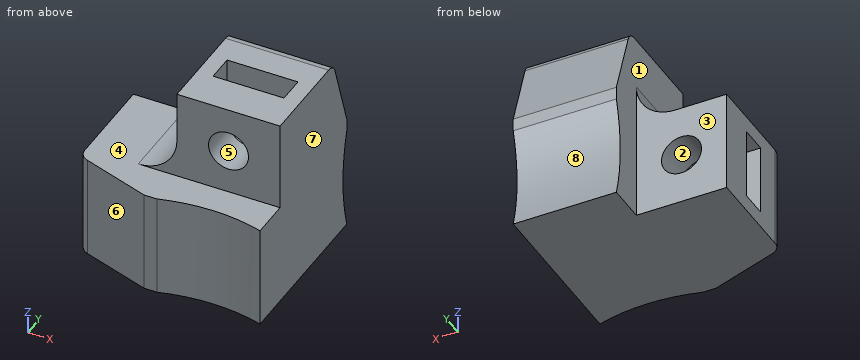
```python
from build123d import *

# Parameters (mm, degrees)
EXTRUDE002_DEPTH                          = 2.1
EXTRUDE002_ONTO_SKETCH006_ROLL_ANGLE      = 90
EXTRUDE001_DEPTH                          = 2.1
EXTRUDE001_ONTO_SKETCH005_ROLL_ANGLE      = 90
EXTRUDE001_ONTO_SKETCH005_PLACEMENT_ANGLE = 180
EXTRUDE_DEPTH                             = 8
SKETCH001_W                               = 8
SKETCH001_H                               = 10
PAD_DEPTH                                 = 7
POCKET_DEPTH                              = 8.001
SKETCH003_R                               = 1.55
POCKET001_DEPTH                           = 7
SKETCH004_R                               = 1.55
POCKET002_DEPTH                           = 7
CHAMFER_SIZE2                             = 2
CHAMFER_SIZE                              = 6
CHAMFER001_SIZE2                          = 6
CHAMFER001_SIZE                           = 2
FILLET_1_R                                = 3
FILLET_2_R                                = 1


with BuildPart() as extrude002:
    # Sketch006 as drawn → Extrude002 (new)
    with BuildSketch(Plane.XY):
        Polygon((4, 8.324574), (1.25, 9.912287), (1.25, 15), (6.75, 15), (6.75, 9.912287), align=None)
    extrude(amount=-EXTRUDE002_DEPTH)


with BuildPart() as extrude002_1:
    # Extrude002 onto Sketch006 roll: moved
    add(extrude002.part.rotate(Axis((0, 0, 0), (1, 0, 0)), EXTRUDE002_ONTO_SKETCH006_ROLL_ANGLE))


with BuildPart() as extrude002_2:
    # Extrude002 onto Sketch006 placement: moved
    add(extrude002_1.part.moved(Location((0, -7, 0))))


with BuildPart() as extrude002_3:
    # Extrude002 placement: moved
    add(extrude002_2.part.moved(Location((0, 3, 0))))


with BuildPart() as extrude001:
    # Sketch005 as drawn → Extrude001 (new)
    with BuildSketch(Plane.XY):
        Polygon((0.324574, 4), (1.912287, 6.75), (7, 6.75), (7, 1.25), (1.912287, 1.25), align=None)
    extrude(amount=-EXTRUDE001_DEPTH)


with BuildPart() as extrude001_1:
    # Extrude001 onto Sketch005 roll: moved
    add(extrude001.part.rotate(Axis((0, 0, 0), (1, 0, 0)), EXTRUDE001_ONTO_SKETCH005_ROLL_ANGLE))


with BuildPart() as extrude001_2:
    # Extrude001 onto Sketch005 placement: moved
    add(extrude001_1.part.rotate(Axis((0, 0, 0), (0, 0, 1)), EXTRUDE001_ONTO_SKETCH005_PLACEMENT_ANGLE))


with BuildPart() as extrude001_3:
    # Extrude001 placement: moved
    add(extrude001_2.part.moved(Location((0, -3, 0))))


with BuildPart() as fillet_body:
    # Sketch → Extrude (new body)
    with BuildSketch(Plane.XY):
        with BuildLine():
            Line((0, 0), (0, 3))
            Line((0, 3), (8, 3))
            Line((8, 3), (8, -10))
            ThreePointArc((8, -10), (4, -9.422859), (0, -10))
            Line((0, -10), (-7, -10))
            Line((-7, -10), (-7, 0))
            Line((-7, 0), (0, 0))
        make_face()
    extrude(amount=EXTRUDE_DEPTH)

    # Sketch001 → Pad (new body)
    with BuildSketch(Plane.XY.offset(8)):
        with Locations((4, -2)):
            Rectangle(SKETCH001_W, SKETCH001_H)
    extrude(amount=PAD_DEPTH)

    # Sketch002 → Pocket (cut, through all)
    with BuildSketch(Plane(origin=(0, 0, 0), x_dir=(0, -1, 0), z_dir=(-1, 0, 0))):
        with BuildLine():
            Line((-3, 0), (-3, 8))
            ThreePointArc((-3, 0), (-2.422859, 4), (-3, 8))
        make_face()
    extrude(amount=-POCKET_DEPTH, mode=Mode.SUBTRACT)

    # Sketch003 → Pocket001 (cut)
    with BuildSketch(Plane(origin=(0, 0, 0), x_dir=(-1, 0, 0), z_dir=(0, 1, 0))):
        with Locations((3.5, 4)):
            Circle(SKETCH003_R)
    extrude(amount=-POCKET001_DEPTH, mode=Mode.SUBTRACT)

    # Sketch004 → Pocket002 (cut)
    with BuildSketch(Plane.XZ.offset(7)):
        with Locations((4, 11.5)):
            Circle(SKETCH004_R)
    extrude(amount=-POCKET002_DEPTH, mode=Mode.SUBTRACT)

    # Cut: cut Extrude001
    add(extrude001_3.part, mode=Mode.SUBTRACT)

    # Cut001: cut Extrude002
    add(extrude002_3.part, mode=Mode.SUBTRACT)

    # Chamfer
    chamfer_edges = [fillet_body.edges().sort_by_distance(p)[0] for p in [
        (4, 3, 15),
    ]]
    chamfer_side = fillet_body.faces().sort_by_distance((4, 3, 11.5))[0]
    chamfer(chamfer_edges, length=CHAMFER_SIZE, length2=CHAMFER_SIZE2, reference=chamfer_side)

    # Chamfer001
    chamfer001_edges = [fillet_body.edges().sort_by_distance(p)[0] for p in [
        (-7, -10, 4),
    ]]
    chamfer001_side = fillet_body.faces().sort_by_distance((-7, -5.160299, 4))[0]
    chamfer(chamfer001_edges, length=CHAMFER001_SIZE, length2=CHAMFER001_SIZE2, reference=chamfer001_side)

    # Fillet 1
    fillet_1_edges = [fillet_body.edges().sort_by_distance(p)[0] for p in [
        (0, -3.5, 8),
    ]]
    fillet(fillet_1_edges, radius=FILLET_1_R)

    # Fillet 2
    fillet_2_edges = [fillet_body.edges().sort_by_distance(p)[0] for p in [
        (-7, -8, 4),
        (4, 1, 15),
    ]]
    fillet(fillet_2_edges, radius=FILLET_2_R)


solid = fillet_body.part
```
The listing builds one solid part. Answer for the finished solid, in the listing's coordinates (mm). Face numbers are marked on the shaded views. A direction names the side the tool comes from. Coordinates: 2 decimals unless noted, no trailing zeros. Loops run counter-clockwise (first coordinate to the right, second up) from the corner with the lowest first, then second, coordinate; pieces in that order, holes last. Notation, with made-up numbers: (-12, -19.5) -> (9, -19.5) arc R36 ccw to (9, 18.5) -> close; hole circle Ø10 at (88, 89). An arc over 180 degrees is marked (long way). Return JSON: item names as keys, results as strings. Group by question number.
(1) Which of the six approach directions +Z, -Z, +X, -X, +Y, -Y give full straight-line access (tool end or side, diameter ignored) to the marked faces 1, 2, 3 and 4?
(2) A cutting plane is placed at D-D on x = 3.5. Write down the section's boundary in (y, z).
(3) Given pin 1 Ø3 at (x, z) = (-2, 4.5) entering from +Y; pin 2 Ø0.9 at (x, z) = (-4, 3.5) entering from +Y; pin 3 Ø4.5 at (x, z) = (4.5, 12.5) entering from -Y, each flat-ended and moving along its own axis, determine where each tip first touches the part or whether it passes through.
(4) Find the intervals of material crossed by probe 1 along Z at (x, y) = (4, -5.4); probe 2 along Z at (x, y) = (-3.5, -5.85); probe 3 along X at (y, z) = (0.5, 14), in increasing order. Write a range as from..to.
(5) A cutting plane is placed at A-A on x = -5.5. Write down the section's boundary in (y, z).
(6) A cutting plane is placed at C-C on z = 4.25. Write down the section's boundary in (x, y), and give its area (3 significant figures).
(7) Determine the mould class of the marked faces 5, 6, 7 and 8 for opening direction X: released by +X, released by -X, zero draft, split by the parting line, or undercut.
(8) A cutting plane is placed at B-B on y = -3.25. Write down the section's boundary in (x, z).
The answers:
{
 "1": {"face 1": "+Z, -X, +Y", "face 2": "+Y", "face 3": "+Z, -Z, -X, +Y", "face 4": "+Z, -X, -Y"},
 "2": {"outline": "(-9.43, 0) -> (3, 0) arc R14.15 cw to (3, 8) -> (3, 9) -> (1.23, 14.32) arc R1 ccw to (0.28, 15) -> (-1.9, 15) -> (-1.9, 12.97) -> (0, 12.97) -> (0, 10.03) -> (-1.9, 10.03) -> (-1.9, 8.61) -> (-4, 8.61) -> (-4, 10.03) -> (-7, 10.03) -> (-7, 8) -> (-9.43, 8) -> close; (-7, 12.97) -> (-4, 12.97) -> (-4, 15) -> (-7, 15) -> close"},
 "3": {"pin 1": "stops at y = 0", "pin 2": "stops at y = -7", "pin 3": "stops at y = -7"},
 "4": {"probe 1": "z = 0..9.95, 13.05..15", "probe 2": "z = 0..2.45, 5.55..8", "probe 3": "x = 0..8"},
 "5": {"outline": "(-8.5, 0) -> (0, 0) -> (0, 8) -> (-8.5, 8) -> close; hole (-5.1, 1.25) -> (-3, 1.25) -> (-3, 6.75) -> (-5.1, 6.75) -> close"},
 "6": {"outline": "(-7, -7.28) arc R1 ccw to (-6.32, -8.23) -> (-1, -10) -> (0, -10) arc R14.15 cw to (8, -10) -> (8, 2.43) -> (0, 2.43) -> (0, 0) -> (-1.97, 0) -> (-1.97, -3) -> (-0.47, -3) -> (-0.47, -5.1) -> (-1.97, -5.1) -> (-1.97, -7) -> (-5.03, -7) -> (-5.03, -5.1) -> (-7, -5.1) -> close; (-7, -3) -> (-5.03, -3) -> (-5.03, 0) -> (-7, 0) -> close", "area": "132 mm^2"},
 "7": {"face 5": "undercut", "face 6": "released by -X", "face 7": "released by +X", "face 8": "zero draft"},
 "8": {"outline": "(-7, 0) -> (8, 0) -> (8, 15) -> (6.75, 15) -> (6.75, 9.91) -> (4, 8.32) -> (1.25, 9.91) -> (1.25, 15) -> (0, 15) -> (0, 11) arc R3 cw to (-3, 8) -> (-7, 8) -> (-7, 6.75) -> (-1.91, 6.75) -> (-0.32, 4) -> (-1.91, 1.25) -> (-7, 1.25) -> close"}
}
